Model file for the job. Use its own axes, mm. Face numbers are marked on the shaded views. A direction names the side the tool comes from. Coordinates: 2 decimals unless noted, no trailing zeros. Order: outer loops, then holes, each group sorted by start corner. A loop starts at its lowest first (then second) coordinate and runs counter-clockwise, first axis right, second up. Notation, with made-up numbers: (55, 9) -> (88, 9) arc R21 ccw to (88, 13) -> close; hole circle Ø4 at (-39, 88). An arc over 180 degrees is marked (long way). Use CSV: the item, a comma, the result in double quotes. Start each with the question number.
(1) Cut at C-C on y = -11. Write the cut outline in (x, z).
(2) Pin check, flat tip, straight feed: pin 1 Ø10 at (x, y) = (-21.5, -20) entering from -Z. Stop position of the tip, or through.
(3) Probe L1, parallel to X at y = -20, z = 2.4; L2, parallel to X at y = -23, z = 1; L3, parallel to Y at x = -16, z = 2.2. List the from-to ranges inside material, lowest first.
(4) Tool access for the marked faces 1 and 2: list every direction of +Z, -Z, +X, -X, +Y, -Y with a clear straight run to the whole face (end or side of a thin tool).
(5) Cut at D-D on x = -15. Write the cut outline in (y, z).
(6) Cut at B-B on x = -20. Write the cut outline in (y, z).
(7) Cut at A-A on z = 1.95. Write the cut outline in (x, y), plus the area to 3 significant figures.
```python
from build123d import *

# Parameters (mm, degrees)
F1_DEPTH = 6
F3_DEPTH = 2.5


with BuildPart() as f1:
    # F0 (on Top) → F1 (new body)
    with BuildSketch(Plane.XY):
        with BuildLine():
            Line((0, -25.719567), (0, 24.280433))
            Line((0, 24.280433), (-40, 24.280433))
            Line((-40, 24.280433), (-40, -25.719567))
            Line((-40, -25.719567), (-23, -25.719567))
            Line((-23, -25.719567), (-23, -21.719567))
            ThreePointArc((-23, -21.719567), (-20, -18.719567), (-17, -21.719567))
            Line((-17, -21.719567), (-17, -25.719567))
            Line((-17, -25.719567), (0, -25.719567))
        make_face()
    extrude(amount=F1_DEPTH)

    # F2 (on face) → F3 (cut)
    with BuildSketch(Plane(origin=(0, 0, 0), x_dir=(1, 0, 0), z_dir=(0, 0, -1))):
        with BuildLine():
            Line((-9.355118, 25.719567), (-30.644882, 25.719567))
            ThreePointArc((-30.644882, 25.719567), (-31.188453, 23.752307), (-31.37161, 21.719567))
            ThreePointArc((-31.37161, 21.719567), (-20, 10.347957), (-8.62839, 21.719567))
            ThreePointArc((-8.62839, 21.719567), (-8.811547, 23.752307), (-9.355118, 25.719567))
        make_face()
        with BuildLine():
            ThreePointArc((-9.355118, 25.719567), (-20, 33.091177), (-30.644882, 25.719567))
            Line((-30.644882, 25.719567), (-9.355118, 25.719567))
        make_face()
        with BuildLine():
            ThreePointArc((-31.37161, 21.719567), (-31.188453, 23.752307), (-30.644882, 25.719567))
            Line((-30.644882, 25.719567), (-31.5, 25.719567))
            Line((-31.5, 25.719567), (-31.37161, 21.719567))
        make_face()
        with BuildLine():
            Line((-8.5, 25.719567), (-9.355118, 25.719567))
            ThreePointArc((-9.355118, 25.719567), (-8.811547, 23.752307), (-8.62839, 21.719567))
            Line((-8.62839, 21.719567), (-8.5, 25.719567))
        make_face()
    extrude(amount=-F3_DEPTH, mode=Mode.SUBTRACT)


solid = f1.part
```
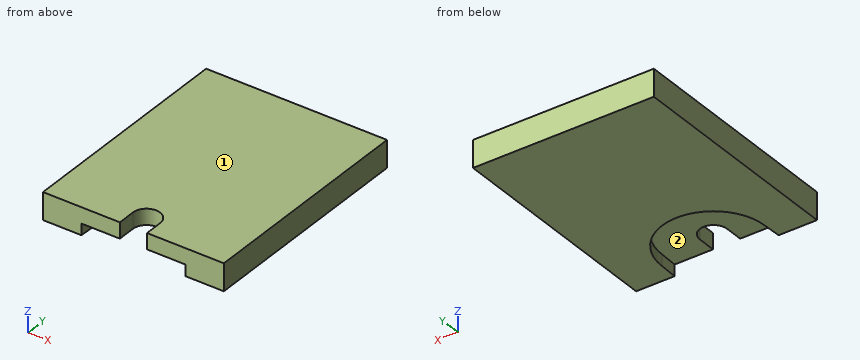
Outcome:
1,outline,"(-40, 0) -> (-23.8, 0) -> (-23.8, 2.5) -> (-16.2, 2.5) -> (-16.2, 0) -> (0, 0) -> (0, 6) -> (-40, 6) -> close"
2,pin 1,"z = 2.5"
3,L1,"-40 to -31.24, -8.76 to 0"
3,L2,"-40 to -31.41, -8.59 to 0"
3,L3,"-11.07 to 24.28"
4,face 1,"+Z, +X, -X, +Y, -Y"
4,face 2,"-Z, -Y"
5,outline,"(-25.72, 2.5) -> (-11.51, 2.5) -> (-11.51, 0) -> (24.28, 0) -> (24.28, 6) -> (-25.72, 6) -> close"
6,outline,"(-18.72, 2.5) -> (-10.35, 2.5) -> (-10.35, 0) -> (24.28, 0) -> (24.28, 6) -> (-18.72, 6) -> close"
7,outline,"(-40, -25.72) -> (-31.5, -25.72) -> (-31.37, -21.72) arc R11.37 cw to (-8.63, -21.72) -> (-8.5, -25.72) -> (0, -25.72) -> (0, 24.28) -> (-40, 24.28) -> close"
7,area,"1,710 mm2"
